Input: part model. Units: mm. Frame: model coordinates. A direction names the side the tool comes from. Coordinates: 2 decimals unless noted, no trailing zeros. Write each loop counter-clockwise with the first axis right and the second up, starting at its lowest first coordinate (ties: lowest second). Pieces come first, ordered by that corner, then holes.
from build123d import *

# Parameters (mm, degrees)
SKETCH3_W                    = 125
SKETCH3_H                    = 70
BASE_FLANGE1_DEPTH           = 2
EDGE_FLANGE2_STRIP_W         = 12
EDGE_FLANGE2_STRIP_H         = 2
EDGE_FLANGE2_STRIP_CUT_DEPTH = 125
EDGE_FLANGE2_DEPTH           = 125
SKETCH18_W                   = 113
SKETCH18_H                   = 52
CUT_EXTRUDE3_DEPTH           = 10
SKETCH23_R                   = 4.5
BOSS_EXTRUDE1_DEPTH          = 2
PSU_BRACKET_MB_HOLES_D       = 3.4
M3_5_CLEARANCE_HOLE1_D       = 3.9


# Sheet-metal steps are written as plain solids
with BuildPart() as part:
    # Sketch3 → Base-Flange1 (new body)
    with BuildSketch(Plane.XY):
        with Locations((-0.781098762, 13.552360409)):
            Rectangle(SKETCH3_W, SKETCH3_H)
    extrude(amount=-BASE_FLANGE1_DEPTH)

    # Edge-Flange2 strip (across the edge) → Edge-Flange2 strip cut (cut)
    with BuildSketch(Plane(origin=(-63.281098762, 48.552360409, -2), x_dir=(0, -1, 0), z_dir=(1, 0, 0))):
        with Locations((-2, -1)):
            Rectangle(EDGE_FLANGE2_STRIP_W, EDGE_FLANGE2_STRIP_H)
    extrude(amount=EDGE_FLANGE2_STRIP_CUT_DEPTH, mode=Mode.SUBTRACT)

    # Edge-Flange2 section (across the edge) → Edge-Flange2 (add)
    with BuildSketch(Plane(origin=(-63.281098762, 48.552360409, -2), x_dir=(0, -1, 0), z_dir=(1, 0, 0))):
        with BuildLine():
            Line((0, 2), (0, 13.7366))
            Line((0, 13.7366), (2, 13.7366))
            Line((2, 13.7366), (2, 2))
            ThreePointArc((2, 2), (2.585786438, 0.585786438), (4, 0))
            Line((4, 0), (4, -2))
            ThreePointArc((4, -2), (1.171572875, -0.828427125), (0, 2))
        make_face()
    extrude(amount=EDGE_FLANGE2_DEPTH)

    # Sketch18 → Cut-Extrude3 (cut)
    with BuildSketch(Plane(origin=(-99.752621101, 247.510324645, -2), x_dir=(1, 0, 0), z_dir=(0, 0, -1))):
        with Locations((98.971522339, 233.957964235)):
            Rectangle(SKETCH18_W, SKETCH18_H)
    extrude(amount=-CUT_EXTRUDE3_DEPTH, mode=Mode.SUBTRACT)

    # Sketch23 → Boss-Extrude1 (add)
    with BuildSketch(Plane.XY):
        with Locations((-57.191455267, 12.802360409)):
            Circle(SKETCH23_R)
        with Locations((-57.191455267, -12.947639591)):
            Circle(SKETCH23_R)
        with Locations((55.718901238, -12.947639591)):
            Circle(SKETCH23_R)
        with Locations((55.718901238, 12.802360409)):
            Circle(SKETCH23_R)
        with Locations((-57.191455267, 38.552360409)):
            Circle(SKETCH23_R)
        with Locations((55.718901238, 38.552360409)):
            Circle(SKETCH23_R)
    extrude(amount=-BOSS_EXTRUDE1_DEPTH)

    # PSU bracket MB holes (through all)
    with Locations(Plane(origin=(-99.752621101, 40.552360409, 598.492474399), x_dir=(1, 0, 0), z_dir=(0, -1, 0))):
        with Locations((43.471522339, -606.610908499), (154.471522339, -606.610908499)):
            Hole(PSU_BRACKET_MB_HOLES_D / 2)

    # M3.5 Clearance Hole1 (through all)
    with Locations(Plane(origin=(-98.752621101, 247.510324645, -2), x_dir=(1, 0, 0), z_dir=(0, 0, -1))):
        with Locations((41.471522339, 260.457964235), (41.471522339, 234.707964235), (41.471522339, 208.957964235), (154.471522339, 208.957964235), (154.471522339, 234.707964235), (154.471522339, 260.457964235)):
            Hole(M3_5_CLEARANCE_HOLE1_D / 2)


solid = part.part
Item 1: Section query B-B, the plane y = 28.5. Return loops of the section in (x, z).
Item 2: Pin query (flat end, axial travel): pin 1 Ø6 at (x, y) = (-57.28, 12.8) entering from -Z; pin 2 Ø1 at (x, z) = (-1.5, -1) entering from +Y; pin 3 Ø6 at (x, z) = (-10, -13.5) entering from -Y; pin 4 Ø3 at (x, y) = (55.72, 38.55) entering from -Z. Return the tip coordinate at first contact, or that it passes through.
Item 3: Section query C-C, the plane z = -5.25. Return loops of the section in (x, y).
Item 4: Section query A-A, the plane x = -40. Return loops of the section in (y, z).
Item 5: Pull-direction query (X, two-part tool) for faces 1 (the face through (53.92, -12.2, -0.99)), 2 (the face through (-2, 46.552, -10)), 3 (the face through (61.719, 21, -1)); classes: released by +X, released by -X, zero draft, split by the parting line, or undercut.
Item 6: Section query D-D, the plane y = 42.5. Return loops of the section in (x, z).
Item 7: Access query for faces 4 (the face through (-54.19, -9.595, -0.986)), 5 (the face through (-1, -13, -2)), 6 (the face through (-2, 48.552, -10)). Directions: +Z, -Z, +X, -X, +Y, -Y. A direction counts if a zero-diameter tool reaches every point of the face in a straight line with its end or side. Return the directions, or none.
Item 8: Material intervals for line 1 (X direction, y = 0.5, z = -1.25); line 2 (Y direction, x = -35, z = -12.5); line 3 (Z direction, x = -36, y = -12.5), sorted ascending.
The answers:
1. outline: (-63.28, -2) - (-57.28, -2) - (-57.28, 0) - (-63.28, 0) - close; (55.72, -2) - (61.72, -2) - (61.72, 0) - (55.72, 0) - close
2. pin 1: stops at z = -2
2. pin 2: stops at y = 47.67
2. pin 3: stops at y = 46.55
2. pin 4: passes through
3. outline: (-63.28, 46.55) - (61.72, 46.55) - (61.72, 48.55) - (-63.28, 48.55) - close
4. outline: (-21.45, -2) - (-12.45, -2) - (-12.45, 0) - (-21.45, 0) - close; (39.55, -2) - (44.55, -2) arc R2 cw to (46.55, -4) - (46.55, -15.74) - (48.55, -15.74) - (48.55, -4) arc R4 ccw to (44.55, 0) - (39.55, 0) - close
5. face 1: undercut
5. face 2: zero draft
5. face 3: released by +X
6. outline: (-63.28, -2) - (61.72, -2) - (61.72, 0) - (-63.28, 0) - close
7. face 4: +Z, -Z
7. face 5: -Z, +X, -X, -Y
7. face 6: +Z, -Z, +X, -X, +Y
8. line 1: x = -63.28 to -57.28, 55.72 to 61.72
8. line 2: y = 46.55 to 48.55
8. line 3: z = -2 to 0
